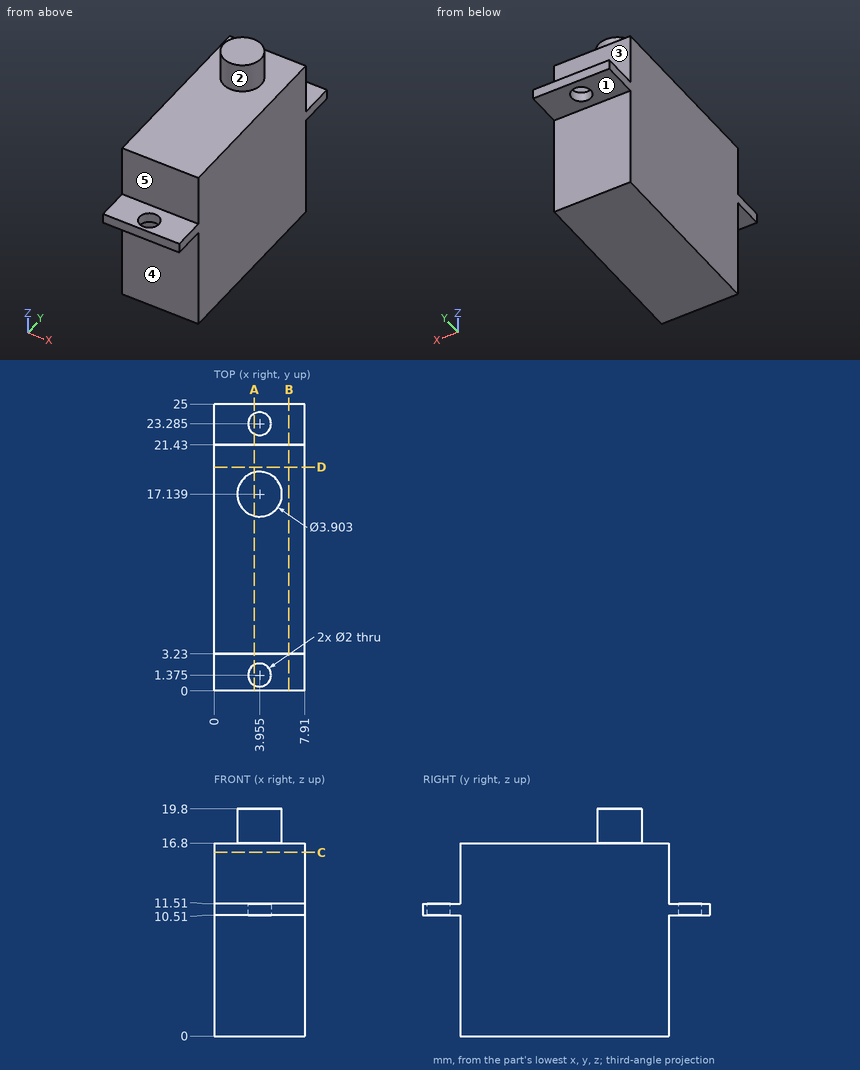
Geometry: see drawing. Coordinates: mm, zero at the bounding-box minimum. A direction names the side the tool comes from. Round coordinates to 2 decimals unless told otherwise and drop trailing zeros. Loops run counter-clockwise (first coordinate to the right, second up) from the corner with the lowest first, then second, coordinate; pieces in that order, holes last. Notation, with made-up numbers: M -20.5,66 L 36.5,66 A30 cw 36.5,99 Z; hole C 68,87.5 d10. An arc over 180 degrees is marked long. Use a Markdown table: item, result. Add a question column.
1. Cut plane A-A, the plane x = 3.5. Output: boundary loops of the cut face in (y, z) (1 decimal), and give its area (3 significant figures).
2. Ray query, line 1 along Y through (x, z) = (2.25, 5); line 2 along Z through (x, y) = (3.25, 14.5); line 3 along Y through (x, z) = (3.5, 11) (1 decimal). Return the intervals inside material, ascending. Write a range as [from, to].
3. Cut plane D-D, the plane y = 19.5. Output: boundary loops of the cut face in (x, z).
4. Cut plane C-C, the plane z = 16. Output: boundary loops of the cut face in (x, y), and give its area (3 significant figures).
5. Contact query for flat-ended pins moving along their axis: pin 1 (1.1 mm diameter, centred on x = 2.5, y = 22.5, fed in from -Z); pin 2 (1.5 mm diameter, centred on x = 6, y = 20, fed in from +Z); pin 3 (4 mm diameter, centred on x = 4, z = 3, fed in from -Y). Output: stop coordinate, or through.
6. Set-up query: the marked faces 1, 2, 3, 4 and 5. Return all of +Z, -Z, +X, -X, +Y, -Y with unobstructed straight access to the full face (end or side cutting, diameter ignored); none if empty.
7. Cut plane B-B, the plane x = 6.5. Output: boundary loops of the cut face in (y, z).
Solution:
| question | item | result |
|---|---|---|
| 1 | outline | M 0,10.5 L 0.5,10.5 L 0.5,11.5 L 0,11.5 Z; M 2.3,10.5 L 3.2,10.5 L 3.2,0 L 21.4,0 L 21.4,10.5 L 22.4,10.5 L 22.4,11.5 L 21.4,11.5 L 21.4,16.8 L 19,16.8 L 19,19.8 L 15.2,19.8 L 15.2,16.8 L 3.2,16.8 L 3.2,11.5 L 2.3,11.5 Z; M 24.2,10.5 L 25,10.5 L 25,11.5 L 24.2,11.5 Z |
| 1 | area | 320 mm2 |
| 2 | line 1 | y = [3.23, 21.43] |
| 2 | line 2 | z = [0, 16.8] |
| 2 | line 3 | y = [0, 0.5], [2.3, 22.4], [24.2, 25] |
| 3 | outline | M 0,0 L 7.91,0 L 7.91,16.8 L 0,16.8 Z |
| 4 | outline | M 0,3.23 L 7.91,3.23 L 7.91,21.43 L 0,21.43 Z |
| 4 | area | 144 mm2 |
| 5 | pin 1 | stops at z = 10.51 |
| 5 | pin 2 | stops at z = 16.8 |
| 5 | pin 3 | stops at y = 3.23 |
| 6 | face 1 | -Z, +X, -X, +Y |
| 6 | face 2 | +Z |
| 6 | face 3 | +Z, +X, -X, +Y |
| 6 | face 4 | -Z, +X, -X, -Y |
| 6 | face 5 | +Z, +X, -X, -Y |
| 7 | outline | M 0,10.51 L 3.23,10.51 L 3.23,0 L 21.43,0 L 21.43,10.51 L 25,10.51 L 25,11.51 L 21.43,11.51 L 21.43,16.8 L 3.23,16.8 L 3.23,11.51 L 0,11.51 Z |
